Build history of the part. All positions in model axes, mm. Face numbers are marked on the shaded views. A direction names the side the tool comes from. Round coordinates to 2 decimals unless told otherwise and drop trailing zeros. Loops run counter-clockwise (first coordinate to the right, second up) from the corner with the lowest first, then second, coordinate; pieces in that order, holes last. Notation, with made-up numbers: (71.5, 53.25) - (122.5, 53.25) arc R27 ccw to (122.5, 74.25) - close; hole circle Ø9 at (73.25, -29). An arc over 180 degrees is marked (long way). Put each result on its own line as item: value. Start each with the question number.
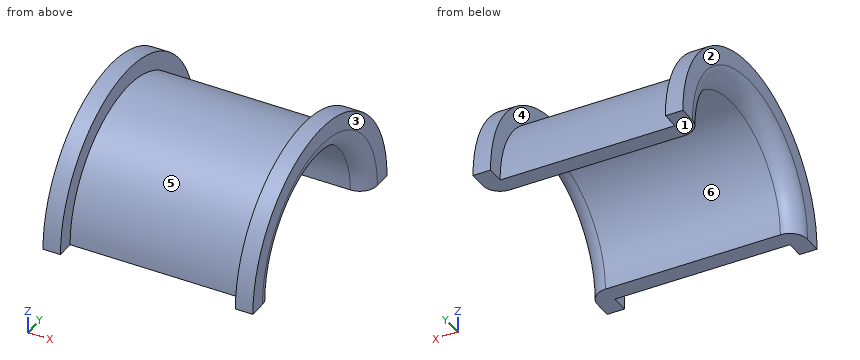
from build123d import *

# Parameters (mm, degrees)
SKETCH1_R               = 30
SKETCH1_R_2             = 25
BOSS_EXTRUDE1_DEPTH     = 25
SKETCH2_R               = 35
SKETCH2_R_2             = 25
BOSS_EXTRUDE2_DEPTH     = 5
FILLET1_R               = 5
CUT_EXTRUDE1_DEPTH      = 78.781745931
CUT_EXTRUDE1_DEPTH_BACK = 78.781745931
SKETCH3_W               = 61.025724242
SKETCH3_H               = 108.223839892


with BuildPart() as part:
    # Sketch1 → Boss-Extrude1 (new, symmetric)
    with BuildSketch(Plane(origin=(0, 0, 0), x_dir=(0, 0, -1), z_dir=(1, 0, 0))):
        Circle(SKETCH1_R)
        Circle(SKETCH1_R_2, mode=Mode.SUBTRACT)
    extrude(amount=BOSS_EXTRUDE1_DEPTH, both=True)

    # Sketch2 → Boss-Extrude2 (add)
    with BuildSketch(Plane(origin=(25, 0, 0), x_dir=(0, 0, -1), z_dir=(1, 0, 0))):
        Circle(SKETCH2_R)
        Circle(SKETCH2_R_2, mode=Mode.SUBTRACT)
    boss_extrude2 = extrude(amount=BOSS_EXTRUDE2_DEPTH)

    # Mirror3: Boss-Extrude2 across plane
    add(boss_extrude2.mirror(Plane(origin=(0, 0, 0), x_dir=(0, 0, 1), z_dir=(1, 0, 0))))

    # Fillet1
    fillet1_edges = [part.edges().sort_by_distance(p)[0] for p in [
        (30, 0, 25),
        (-30, 0, 25),
    ]]
    fillet(fillet1_edges, radius=FILLET1_R - 0.0001)  # a hair under: the kernel refuses the full size

    # Sketch3 → Cut-Extrude1 (cut, two sides: drawn at the far end of the back side and taken through both)
    with BuildSketch(Plane(origin=(30, 0, 0), x_dir=(0, 0, -1), z_dir=(1, 0, 0)).offset(-CUT_EXTRUDE1_DEPTH_BACK)):
        with Locations((30.512862121, 2.693719616)):
            Rectangle(SKETCH3_W, SKETCH3_H)
    extrude(amount=CUT_EXTRUDE1_DEPTH + CUT_EXTRUDE1_DEPTH_BACK, mode=Mode.SUBTRACT)


solid = part.part
Item 1: Which spindle directions (+Z, -Z, +X, -X, +Y, -Y) get a long thin tool onto all of the face, cutting with end or side? Do the marked faces 5 and 6. Say none if no direction does.
Item 2: Two-plate mould, pull along X, no slides. Class the marked faces 1, 2, 3 and 4: pulls with the +X half, pulls with the -X half, needs draft (parallel to the pull), parting line crosses it, or undercut.
Item 3: Drill centre lines: probe 1 along X at (y, z) = (-5, 32.5); probe 2 along Y at (x, z) = (-14, 7); probe 3 along Y at (x, z) = (-10, 10). Where is each one in solid material? Low to high. Write a range as [from, to].
Item 4: Slice it at B-B (z = 31). Give the cut face in (x, y), plus the area to 3 significant figures.
Item 5: Slice it at C-C (x = -14). Give the cut face in (y, z), plus the area to 3 significant figures.
Item 6: Slice it at A-A (y = 0). Give the cut face in (x, z), plus the area to 3 significant figures.
Item 7: Drop flat-ended pins along their axis: pin 1 Ø6 at (x, z) = (5.5, 4) entering from +Y; pin 2 Ø1.5 at (y, z) = (-21.5, 9) entering from +X (3 decimals); pin 3 Ø3 at (x, z) = (-8, 17) entering from -Y; pin 4 Ø1 at (y, z) = (27, 3.5) entering from +X. Give the stop position or say it passes through.
Computed values:
1. face 5: +Z
1. face 6: -Z, +X, -X
2. face 1: needs draft
2. face 2: pulls with the -X half
2. face 3: pulls with the +X half
2. face 4: undercut
3. probe 1: x = [-30, -25], [25, 30]
3. probe 2: y = [-29.17, -24], [24, 29.17]
3. probe 3: y = [-28.28, -22.91], [22.91, 28.28]
4. outline: (-30, -16.25) - (-25, -16.25) - (-25, 16.25) - (-30, 16.25) - close; (25, -16.25) - (30, -16.25) - (30, 16.25) - (25, 16.25) - close
4. area: 325 mm^2
5. outline: (-30, 0) - (-25, 0) arc R25 cw to (25, 0) - (30, 0) arc R30 ccw to start
5. area: 432 mm^2
6. outline: (-30, 30) arc R5 ccw to (-25, 25) - (25, 25) arc R5 ccw to (30, 30) - (30, 35) - (25, 35) - (25, 30) - (-25, 30) - (-25, 35) - (-30, 35) - close
6. area: 339 mm^2
7. pin 1: stops at y = 29.98
7. pin 2: passes through
7. pin 3: stops at y = -25.69
7. pin 4: stops at x = 29.45
